from build123d import *

# Parameters (mm, degrees)
ESQUISSE1_W             = 7.5
ESQUISSE1_H             = 7.5
BOSS_EXTRU_1_DEPTH      = 65
ESQUISSE2_R             = 1.25
ENL_V_MAT_EXTRU_1_DEPTH = 66.538633645
ENL_V_START             = -30
ENL_V_MAT_EXTRU_2_DEPTH = 36.215987304
CONG_1_R                = 1.5


with BuildPart() as part:
    # Esquisse1 → Boss.-Extru.1 (new body)
    with BuildSketch(Plane.XY):
        Rectangle(ESQUISSE1_W, ESQUISSE1_H)
    extrude(amount=BOSS_EXTRU_1_DEPTH)

    # Esquisse2 → Enlèv. mat.-Extru.1 (cut, through all)
    with BuildSketch(Plane(origin=(0, 3.75, 0), x_dir=(1, 0, 0), z_dir=(0, 1, 0))):
        with Locations(Location((0, -4.5, 0), (0, 0, 270))):
            Circle(ESQUISSE2_R)
        with Locations(Location((0, -25.5, 0), (0, 0, 270))):
            Circle(ESQUISSE2_R)
    extrude(amount=-ENL_V_MAT_EXTRU_1_DEPTH, mode=Mode.SUBTRACT)

    # Esquisse3 → Enlèv. mat.-Extru.2 (cut, through all)
    with BuildSketch(Plane(origin=(0, 0, 0), x_dir=(-1, 0, 0), z_dir=(0, 0, -1)).offset(ENL_V_START)):
        Polygon((-1.25, 3.75), (-3.75, 3.75), (-3.75, 1.25), align=None)
        Polygon((-3.75, -1.25), (-3.75, -3.75), (-1.25, -3.75), align=None)
    extrude(amount=-ENL_V_MAT_EXTRU_2_DEPTH, mode=Mode.SUBTRACT)

    # Congé1
    cong_1_edges = [part.edges().sort_by_distance(p)[0] for p in [
        (2.5, 2.5, 30),
        (2.5, -2.5, 30),
    ]]
    fillet(cong_1_edges, radius=CONG_1_R)


solid = part.part
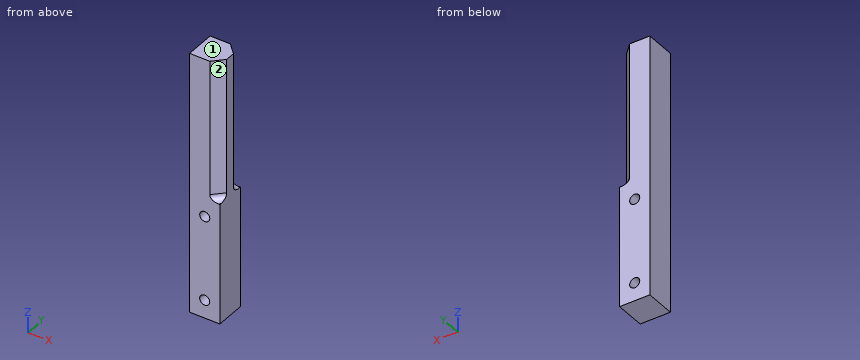
Could you check a few things on this model? Use its own coordinates, in mm. Face numbers are marked on the shaded views. A direction names the side the tool comes from. Coordinates: 2 decimals unless noted, no trailing zeros. Loops run counter-clockwise (first coordinate to the right, second up) from the corner with the lowest first, then second, coordinate; pieces in that order, holes last.
1. For the marked faces 1 and 2, which set-ups out of +Z, -Z, +X, -X, +Y, -Y let a thin tool reach every point of the face, with its end or its side?
2. Imagine slicing it at A-A (z = 25.5). Please give me the cut outline in (x, y), and give its area (3 significant figures).
3. Imagine slicing it at C-C (y = -0.5). Please give me the cut outline in (x, z).
4. Imagine slicing it at D-D (z = 36.5). Please give me the cut outline in (x, y), and give its area (3 significant figures).
5. I need wall thicknesses on L1, parallel to X at y = 2, z = 4.5; L2, parallel to X at y = -1.25, z = 4; L3, parallel to Y at x = 2.25, z = 58. Which ranges of each line are inside material? Lowest first, please.
6. Imagine slicing it at B-B (x = 0). Please give me the cut outline in (y, z), and give its area (3 significant figures).
Computed values:
1. face 1: +Z, +X, -X, +Y, -Y
1. face 2: +Z, +X, -Y
2. outline: (-3.75, -3.75) - (-1.25, -3.75) - (-1.25, 3.75) - (-3.75, 3.75) - close; (1.25, -3.75) - (3.75, -3.75) - (3.75, 3.75) - (1.25, 3.75) - close
2. area: 37.5 mm2
3. outline: (-3.75, 0) - (3.75, 0) - (3.75, 65) - (-3.75, 65) - close; hole circle Ø2.5 at (0, 4.5); hole circle Ø2.5 at (0, 25.5)
4. outline: (-3.75, -3.75) - (1.25, -3.75) - (3.75, -1.25) - (3.75, 1.25) - (1.25, 3.75) - (-3.75, 3.75) - close
4. area: 50.0 mm2
5. L1: x = -3.75 to -1.25, 1.25 to 3.75
5. L2: x = -3.75 to -1.15, 1.15 to 3.75
5. L3: y = -2.75 to 2.75
6. outline: (-3.75, 0) - (3.75, 0) - (3.75, 3.25) - (-3.75, 3.25) - close; (-3.75, 5.75) - (3.75, 5.75) - (3.75, 24.25) - (-3.75, 24.25) - close; (-3.75, 26.75) - (3.75, 26.75) - (3.75, 65) - (-3.75, 65) - close
6. area: 450 mm2
